Can you work these out from the model? Positions are in its coordinate system, mm. Face numbers are marked on the shaded views. A direction names the side the tool comes from. Coordinates: 2 decimals unless noted, no trailing zeros. Order: outer loops, then holes, each group sorted by start corner. A loop starts at its lowest first (then second) coordinate and runs counter-clockwise, first axis right, second up. Notation, with made-up numbers: M 14,82 L 30,82 A24 cw 30,111 Z; hole C -23.75,-27 d11. An arc over 180 degrees is marked long. Answer as CSV lines item,"result". Start each with the question number.
1. If we section it at B-B (z = -49): List the corners of the cut face in (x, y) for me.
2. If we section it at C-C (x = 10): List the corners of the cut face in (y, z) for me.
3. Will these pins go through, and if not, where does the flat tip stop? pin 1 (1.5 mm diameter, centred on y = 5.5, z = -65.5, fed in from +X); pin 2 (0.9 mm diameter, centred on x = 35.5, y = 4.5, fed in from -Z); pin 3 (2 mm diameter, centred on x = 11.5, y = 0.5, fed in from +Z); pin 4 (1.2 mm diameter, centred on y = 1, z = -133, fed in from +X).
4. I need wall thicknesses on line 1 along X through (y, z) = (5.5, -21.5); line 2 along Y through (x, z) = (-10, -38); line 3 along Z through (x, y) = (43.5, 4.25). Which ranges of each line are inside material? Lowest first, please. Write a range as from..to.
5. On a 3-axis mill with a long thin cutter (end or side, diameter ignored), from which of +Z, -Z, +X, -X, +Y, -Y can I reach the whole of each face in a straight line? I mean the marked faces 1 and 2. Say none if no direction works.
6. If we section it at A-A (x = -18): List the corners of the cut face in (y, z) for me.
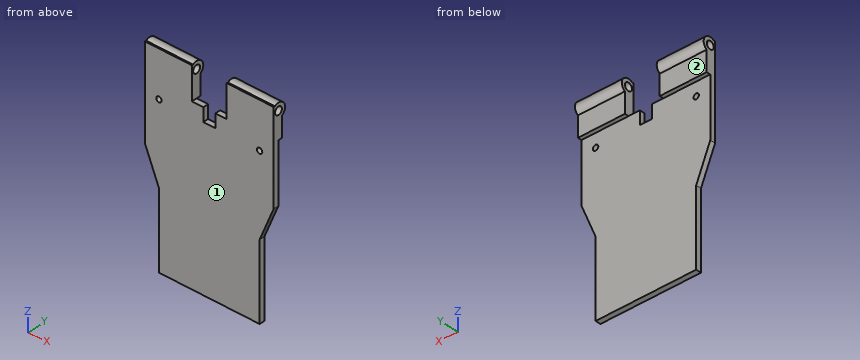
```python
from build123d import *

# Parameters (mm, degrees)
BOSS_EXTRUDE1_DEPTH = 3
SKETCH5_W           = 35
SKETCH5_H           = 23
BOSS_EXTRUDE2_DEPTH = 3
BOSS_EXTRUDE5_DEPTH = 35
BOSS_EXTRUDE8_START = -35
BOSS_EXTRUDE8_DEPTH = 35
CUT_EXTRUDE1_START  = -96
SKETCH11_R          = 2.9
CUT_EXTRUDE1_DEPTH  = 96
BOSS_EXTRUDE7_DEPTH = 1
SKETCH17_R          = 2
CUT_EXTRUDE2_DEPTH  = 10


with BuildPart() as part:
    # Sketch1 → Boss-Extrude1 (new body)
    with BuildSketch(Plane(origin=(0, 0, 0), x_dir=(1, 0, 0), z_dir=(0, 1, 0))):
        Polygon((0, 0), (0, 23), (8.5, 23), (8.5, 33), (17.5, 33), (17.5, 23), (26, 23), (26, 0), (61, 0), (61, 28.801365462), (61, 67.406151765), (50.5, 93.029580251), (50.5, 150), (-24.5, 150), (-24.5, 93.029580251), (-35, 67.406151765), (-35, 28.801365462), (-35, 0), align=None)
    extrude(amount=BOSS_EXTRUDE1_DEPTH)

    # Sketch5 → Boss-Extrude2 (add)
    with BuildSketch(Plane(origin=(0, 3, 0), x_dir=(1, 0, 0), z_dir=(0, 1, 0))):
        with Locations((-17.5, 11.5)):
            Rectangle(SKETCH5_W, SKETCH5_H)
        with Locations((43.5, 11.5)):
            Rectangle(SKETCH5_W, SKETCH5_H)
    extrude(amount=BOSS_EXTRUDE2_DEPTH)

    # Sketch12 → Boss-Extrude5 (add)
    with BuildSketch(Plane.ZY.offset(35)):
        with BuildLine():
            Line((-7.857598958, 0), (1.361945499, 0))
            ThreePointArc((1.361945499, 0), (-3.247826729, 8.5), (-7.857598958, 0))
        make_face()
    extrude(amount=-BOSS_EXTRUDE5_DEPTH)

    # Sketch15 → Boss-Extrude8 (add)
    with BuildSketch(Plane(origin=(61, 0, 0), x_dir=(0, 0, -1), z_dir=(1, 0, 0)).offset(BOSS_EXTRUDE8_START)):
        with BuildLine():
            Line((7.857598958, 0), (-1.361945499, 0))
            ThreePointArc((-1.361945499, 0), (3.247826729, 8.5), (7.857598958, 0))
        make_face()
    extrude(amount=BOSS_EXTRUDE8_DEPTH)

    # Sketch11 → Cut-Extrude1 (cut)
    with BuildSketch(Plane.ZY.offset(35).offset(CUT_EXTRUDE1_START)):
        with Locations((-3.247826729, 3)):
            Circle(SKETCH11_R)
    extrude(amount=CUT_EXTRUDE1_DEPTH, mode=Mode.SUBTRACT)

    # Sketch14 → Boss-Extrude7 (add)
    with BuildSketch(Plane.XZ):
        Polygon((50.5, -93.029580251), (61, -67.406151765), (61, 1.361945499), (26, 1.361945499), (26, -23), (17.5, -23), (17.5, -33), (8.5, -33), (8.5, -23), (0, -23), (0, 1.361945499), (-35, 1.361945499), (-35, -67.406151765), (-24.5, -93.029580251), (-24.5, -150), (50.5, -150), align=None)
    extrude(amount=BOSS_EXTRUDE7_DEPTH)

    # Sketch17 → Cut-Extrude2 (cut)
    with BuildSketch(Plane(origin=(0, 3, 0), x_dir=(1, 0, 0), z_dir=(0, 1, 0))):
        with Locations(Location((-24.5, 33, 0), (0, 0, 270))):
            Circle(SKETCH17_R)
        with Locations(Location((50.5, 33, 0), (0, 0, 270))):
            Circle(SKETCH17_R)
    extrude(amount=-CUT_EXTRUDE2_DEPTH, mode=Mode.SUBTRACT)


solid = part.part
```
Solved:
1,outline,"M -35,-1 L 61,-1 L 61,3 L -35,3 Z"
2,outline,"M -1,-150 L 3,-150 L 3,-33 L -1,-33 Z"
3,pin 1,"through"
3,pin 2,"z = -23"
3,pin 3,"z = -33"
3,pin 4,"x = 50.5"
4,line 1,"-35..0, 26..61"
4,line 2,"-1..3"
4,line 3,"-23..-5.86, -0.63..2.11"
5,face 1,"+Z, -Z, +X, -X, -Y"
5,face 2,"-Z, +X, -X, +Y"
6,outline,"M -1,-150 L 3,-150 L 3,-23 L 6,-23 L 6,-7.86 A5.5 ccw 0,1.36 L -1,1.36 Z; hole C 3,-3.25 d5.8"
